Model file for the job. Use its own axes, mm. A direction names the side the tool comes from. Coordinates: 2 decimals unless noted, no trailing zeros. Loops run counter-clockwise (first coordinate to the right, second up) from the corner with the lowest first, then second, coordinate; pieces in that order, holes last. Notation, with made-up numbers: M 70.25,60 L 127.25,60 A14 cw 127.25,78 Z; hole C 65.5,30.5 d10. An arc over 180 degrees is marked long. Write item = value, one per line. Start each with the question number.
Autodesk Inventor part; units mm, degrees
ref_plane "Work Plane1" through (-0.719, -0.719, -11.9062) normal (-0.7071, -0.7071, 0) x (0.7071, -0.7071, 0)
ref_plane "YZ Plane" through (0, 0, 0) normal (1, 0, 0) x (0, 1, 0)
ref_plane "XZ Plane" through (0, 0, 0) normal (0, 1, 0) x (-1, 0, 0)
sketch "Sketch1" plane through (0, 0, 0) normal (0, 0, 1) x (1, 0, 0)
  line L0 (-76.2, 76.2) -> (76.2, 76.2) construction
  line L1 (76.2, 76.2) -> (76.2, -76.2) construction
  line L2 (76.2, -76.2) -> (-76.2, -76.2) construction
  line L3 (-76.2, -76.2) -> (-76.2, 76.2) construction
  line L4 (-76.2, 76.2) -> (76.2, -76.2) construction
  line L5 (76.2, 76.2) -> (-76.2, -76.2) construction
  circle A0 centre (-76.2, -76.2) radius 16.764 construction
  circle A1 centre (76.2, -76.2) radius 16.764 construction
  circle A2 centre (-19.05, -19.05) radius 8.7313
  circle A3 centre (19.05, -19.05) radius 8.7313 construction
  line L6 (-19.05, -19.05) -> (19.05, -19.05) construction
  circle A4 centre (-19.05, -19.05) radius 19.05 construction
  circle A5 centre (19.05, -19.05) radius 19.05 construction
  circle A6 centre (-19.05, -19.05) radius 18.796 construction
  circle A7 centre (19.05, -19.05) radius 18.796 construction
  arc A8 (-59.436, -76.2) -> (-76.2, -59.436) centre (-76.2, -76.2) ccw
  line L7 (-19.05, 0) -> (-3.4943, 0)
  line L8 (-33.6217, -7.1775) -> (-76.2, -59.436)
  line L9 (-7.1775, -33.6217) -> (-59.436, -76.2)
  line L10 (-19.05, -0.254) -> (-0.254, -0.254)
  line L11 (-0.254, -0.254) -> (-0.254, -19.05)
  arc A9 (-19.05, -0.254) -> (-33.6217, -7.1775) centre (-19.05, -19.05) ccw
  arc A10 (-7.1775, -33.6217) -> (-0.254, -19.05) centre (-19.05, -19.05) ccw
  point P0 (0, 0)
  point P1 (-33.1106, -7.4056)
  dimension "d0" = 152.4
  dimension "d1" = 152.4
  dimension "d2" = 33.528
  dimension "d3" = 17.4625
  dimension "d4" = 38.1
  dimension "d7" = 0.254
  dimension "d8" = 0.254
extrude "Extrusion1" add sketch "Sketch1" along normal mid plane 23.8125
fillet "Fillet1" radius 1.5875 3 edges at (-0.254, -0.254, 0) (-76.2, -59.436, 0) (-59.436, -76.2, 0)
sketch "Sketch2" plane through (0, 0, 11.9062) normal (0, 0, 1) x (1, 0, 0)
  circle A0 centre (-19.05, -19.05) radius 8.7312
  circle A1 centre (-19.05, -19.05) radius 14.2875
  point P0 (0, 0)
  dimension "d12" = 28.575
extrude "Extrusion2" [suppressed]
mirror "Mirror1" [suppressed]
sketch "Sketch3" plane through (0, 0, 11.9062) normal (0, 0, 1) x (1, 0, 0)
  arc A0 (-59.6805, -73.3471) -> (-57.1134, -74.3077) centre (-58.1162, -73.077) ccw construction
  line L0 (-57.1134, -74.3077) -> (-7.1775, -33.6217) construction
  arc A1 (-7.1775, -33.6217) -> (-0.254, -19.05) centre (-19.05, -19.05) ccw construction
  line L1 (-0.254, -19.05) -> (-0.254, -1.8415) construction
  arc A2 (-0.254, -1.8415) -> (-1.8415, -0.254) centre (-1.8415, -1.8415) ccw construction
  line L2 (-1.8415, -0.254) -> (-19.05, -0.254) construction
  arc A3 (-19.05, -0.254) -> (-33.6217, -7.1775) centre (-19.05, -19.05) ccw construction
  line L3 (-33.6217, -7.1775) -> (-74.3077, -57.1134) construction
  arc A4 (-74.3077, -57.1134) -> (-73.3471, -59.6805) centre (-73.077, -58.1162) ccw construction
  arc A5 (-59.6805, -73.3471) -> (-73.3471, -59.6805) centre (-76.2, -76.2) ccw construction
  line L4 (19.05, 0) -> (-21.3612, -40.4112) construction
  line L5 (19.05, 0) -> (-21.3612, 40.4112) construction
  line L6 (19.05, 0) -> (0, 0) construction
  point P0 (-6.35, 0)
  dimension "d15" = 6.096
  dimension "d17" = 25.4
  dimension "d18" = 57.15
  dimension "d19" = 57.15
  dimension "d20" = 45
ref_plane "Work Plane1" through (-0.719, -0.719, -11.9062) normal (-0.7071, -0.7071, 0) x (0.7071, -0.7071, 0)
sketch "Sketch5" plane through (-19.05, -0.254, 11.9062) normal (0, 1, 0) x (1, 0, 0)
  line L0 (18.796, 0) -> (18.796, 23.8125) construction
  line L1 (-14.5717, 0) -> (-14.5717, 23.8125) construction
  circle A0 centre (3.556, 11.9062) radius 2.875
  point P0 (19.05, 11.9062)
  point P1 (-14.5717, 11.9062)
  dimension "d28" = 15.24
  dimension "d29" = 5.75
extrude "Extrusion3" cut sketch "Sketch5" against normal blind 7.62
equation "\"d7\" = d8"
equation "\"d19\" = d18"
properties part number "CL7-004" material "ABS Plastic"
Item 1: Pull direction X, two halves, no side cores. Call faces 1 (the cylindrical face through (-17.613, -4.011, -1.943)), 2 (the cylindrical face through (-27.222, -2.123, -0.167)), 3 (the flat face through (-38, -37, 11.906)): +X half, -X half, draft (parallel to the pull), parting line (faces both ways), or undercut.
Item 2: Cut at B-B (y = -11.5). Give the cut face in (x, z), plus the area to 3 significant figures.
Item 3: Probe L1, parallel to X at y = -23.5, z = 10.75; L2, parallel to X at y = -3.25, z = 0; L3, parallel to Y at x = -12, z = -6. List the from-to ranges inside material, lowest first.
Item 4: Cut at D-D (x = -55). Give the cut face in (y, z), plus the area to 3 significant figures.
Item 5: 3-axis set-ups, long thin cutter, end or side, ignore diameter. For faces 4 (the flat face through (-16, -7.874, 0)), 5 (the flat face through (-31.796, -53.68, -0.167)): which of +Z, -Z, +X, -X, +Y, -Y reach the whole face in a straight line?
Item 6: Pin check, flat tips, straight feed: pin 1 Ø5 at (x, z) = (-21, 8.5) entering from +Y; pin 2 Ø5 at (x, z) = (-15.494, 0) entering from +Y; pin 3 Ø10 at (x, z) = (-25.5, -9) entering from -Y; pin 4 Ø2 at (x, z) = (-27, -3.5) entering from -Y. Stop position of each tip, or through.
Reported:
q1.face_1 = undercut
q1.face_2 = -X half
q1.face_3 = draft
q2.outline = M -37.14,-11.91 L -23.44,-11.91 L -23.44,11.91 L -37.14,11.91 Z; M -14.66,-11.91 L -0.25,-11.91 L -0.25,11.91 L -14.66,11.91 Z
q2.area = 670 mm^2
q3.L1 = -46.92 to -26.56, -11.54 to -0.79
q3.L2 = -29.23 to -18.37, -12.62 to -0.25
q3.L3 = -37.55 to -24.2, -13.9 to -0.25
q4.outline = M -72.59,-11.91 L -33.42,-11.91 L -33.42,11.91 L -72.59,11.91 Z
q4.area = 933 mm^2
q5.face_4 = +Y
q5.face_5 = +Z, -Z, +X, -Y
q6.pin_1 = -0.25
q6.pin_2 = -7.87
q6.pin_3 = -52.62
q6.pin_4 = -50.59
